CAD build for the part. Positions are in the model's coordinates, mm. Coordinates: 2 decimals unless noted, no trailing zeros. Order: outer loops, then holes, each group sorted by start corner. A loop starts at its lowest first (then second) coordinate and runs counter-clockwise, first axis right, second up. Notation, with made-up numbers: M 75,-12.5 L 112,-12.5 A22 cw 112,26.5 Z; hole C -30.75,-37 d11. An arc over 180 degrees is marked long. Write item = value, one per line.
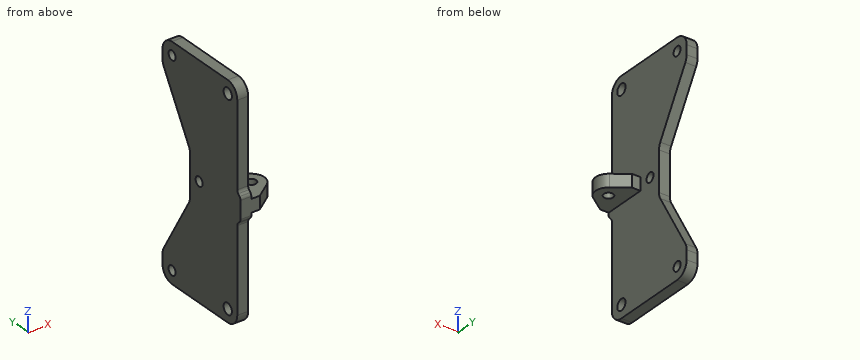
Autodesk Inventor part; units mm, degrees
ref_plane "YZ Plane" through (0, 0, 0) normal (1, 0, 0) x (0, 1, 0)
ref_plane "XZ Plane" through (0, 0, 0) normal (0, 1, 0) x (-1, 0, 0)
ref_plane "XY Plane" through (0, 0, 0) normal (0, 0, 1) x (1, 0, 0)
sketch "Sketch1" plane through (0, 0, 0) normal (1, 0, 0) x (0, 1, 0)
  circle A0 centre (45, 0) radius 11
  line L0 (45, 0) -> (0, 0)
  circle A1 centre (130, 235) radius 11
  line L1 (73.2002, 0) -> (73.2002, 46.6199)
  line L2 (77.2194, 61.6199) -> (155.9808, 198.0385)
  line L3 (160, 213.0385) -> (160, 235)
  arc A2 (160, 235) -> (130, 265) centre (130, 235) ccw
  line L4 (130, 235) -> (130, 265) construction
  line L5 (130, 235) -> (160, 235) construction
  line L6 (130, 265) -> (-45, 265)
  line L7 (0, 0) -> (0, 265)
  circle A3 centre (-45, 235) radius 13
  arc A4 (-45, 265) -> (-75, 235) centre (-45, 235) ccw
  line L8 (-45, 235) -> (-75, 235) construction
  line L9 (-45, 235) -> (-45, 265) construction
  line L10 (-75, 235) -> (-75, 39.1421)
  line L11 (0, 0) -> (-45, 0)
  circle A5 centre (130, -235) radius 11
  line L12 (73.2002, 0) -> (73.2002, -46.6199)
  line L13 (77.2194, -61.6199) -> (155.9808, -198.0385)
  line L14 (160, -213.0385) -> (160, -235)
  arc A6 (130, -265) -> (160, -235) centre (130, -235) ccw
  line L15 (130, -265) -> (-45, -265)
  circle A7 centre (-45, -235) radius 13
  arc A8 (-75, -235) -> (-45, -265) centre (-45, -235) ccw
  line L16 (-45, -235) -> (-75, -235) construction
  line L17 (-75, -235) -> (-75, -39.1421)
  arc A9 (155.9808, 198.0385) -> (160, 213.0385) centre (130, 213.0385) ccw
  arc A10 (77.2194, 61.6199) -> (73.2002, 46.6199) centre (103.2002, 46.6199) ccw
  arc A11 (73.2002, -46.6199) -> (77.2194, -61.6199) centre (103.2002, -46.6199) ccw
  arc A12 (160, -213.0385) -> (155.9808, -198.0385) centre (130, -213.0385) ccw
  line L18 (-77.9289, 32.0711) -> (-82.0711, 27.9289)
  line L19 (-85, 20.8579) -> (-85, 0)
  line L20 (-77.9289, -32.0711) -> (-82.0711, -27.9289)
  line L21 (-85, -20.8579) -> (-85, 0)
  arc A13 (-77.9289, 32.0711) -> (-75, 39.1421) centre (-85, 39.1421) ccw
  arc A14 (-82.0711, 27.9289) -> (-85, 20.8579) centre (-75, 20.8579) ccw
  arc A15 (-85, -20.8579) -> (-82.0711, -27.9289) centre (-75, -20.8579) ccw
  arc A16 (-75, -39.1421) -> (-77.9289, -32.0711) centre (-85, -39.1421) ccw
  point P0 (73.2002, 54.6584)
  point P1 (160, 205)
  point P2 (-75, -35)
  point P3 (48.2002, -10.5242)
  point P4 (73.2002, -54.6584)
  point P5 (160, -205)
  point P6 (-85, 25)
  point P7 (-75, 35)
  point P8 (-85, -25)
  dimension "d0" = 22
  dimension "d1" = 22
  dimension "d2" = 470
  dimension "d3" = 90
  dimension "d7" = 30
  dimension "d8" = 26
  dimension "d9" = 90
  dimension "d11" = 25
  dimension "d12" = 85
  dimension "d13" = 90
  dimension "d14" = 30
  dimension "d15" = 30
  dimension "d16" = 30
  dimension "d19" = 45
  dimension "d20" = 40
  dimension "d21" = 50
  dimension "d22" = 10
extrude "Extrusion1" add sketch "Sketch1" along normal mid plane 25.4
sketch "Sketch2" plane through (0, 0, 0) normal (0, 0, 1) x (1, 0, 0)
  line L0 (12.7, -45) -> (12.7, 130)
  line L1 (12.7, -85) -> (12.7, -82.0711)
  line L2 (12.7, -85) -> (12.7, 15)
  circle A0 centre (50.3463, -35) radius 11
  line L3 (12.7, 15) -> (32.5059, 15)
  line L4 (32.5059, 15) -> (53.1062, 15) construction
  arc A1 (66.6123, -60.2075) -> (66.6123, -9.7925) centre (50.3463, -35) ccw
  line L5 (66.6123, -9.7925) -> (32.5059, 15)
  line L6 (66.6123, -60.2075) -> (32.5059, -85)
  line L7 (32.5059, -85) -> (12.7, -85)
  point P0 (0, 0)
  dimension "d23" = 100
  dimension "d24" = 22
  dimension "d26" = 60
extrude "Extrusion2" add sketch "Sketch2" along normal mid plane 30
properties part number "Balancim_3-Cabos_Modelo2"
(1) Slice it at A-A, the plane z = 0. Write the cut outline in (x, y).
Evaluation:
outline = M -12.7,-85 L 32.51,-85 L 66.61,-60.21 A30 ccw 66.61,-9.79 L 32.51,15 L 12.7,15 L 12.7,34 L -12.7,34 Z; M -12.7,56 L 12.7,56 L 12.7,73.2 L -12.7,73.2 Z; hole C 50.35,-35 d22
(2) Pin check, flat tips, straight feed: pin 1 Ø3 at (x, z) = (62, -2) entering from +Y; pin 2 Ø1.5 at (y, z) = (2, 211.5) entering from +X; pin 3 Ø12.5 at (x, z) = (4.5, -98.5) entering from -Y. Stop position of each tip, or through.
Evaluation:
pin_1 = -5.35
pin_2 = 12.7
pin_3 = -75
(3) Slice it at D-D, the plane x = 27. Write the cut outline in (y, z), then the cut area to 3 significant figures.
Evaluation:
outline = M -85,-15 L 15,-15 L 15,15 L -85,15 Z
area = 3,000 mm²
(4) Slice it at B-B, the plane x = 54.5. Write the cut outline in (y, z), then the cut area to 3 significant figures.
Evaluation:
outline = M -69.01,-15 L -45.19,-15 L -45.19,15 L -69.01,15 Z; M -24.81,-15 L -0.99,-15 L -0.99,15 L -24.81,15 Z
area = 1,430 mm²
(5) Wall check: line 1 (Z direction, x = 1, y = -45); line 2 (Z direction, x = 1.75, y = 45); line 3 (Z direction, x = 0, y = 130). Give the ranges that are in metal, low to high. Write a range as from..to.
Evaluation:
line_1 = -265..-248, -222..222, 248..265
line_2 = -265..-11, 11..265
line_3 = -265..-246, -224..-153.04, 153.04..224, 246..265
(6) Slice it at C-C, the plane y = 125. Write the cut outline in (x, z), then the cut area to 3 significant figures.
Evaluation:
outline = M -12.7,-265 L 12.7,-265 L 12.7,-244.8 L -12.7,-244.8 Z; M -12.7,-225.2 L 12.7,-225.2 L 12.7,-144.38 L -12.7,-144.38 Z; M -12.7,144.38 L 12.7,144.38 L 12.7,225.2 L -12.7,225.2 Z; M -12.7,244.8 L 12.7,244.8 L 12.7,265 L -12.7,265 Z
area = 5,130 mm²
